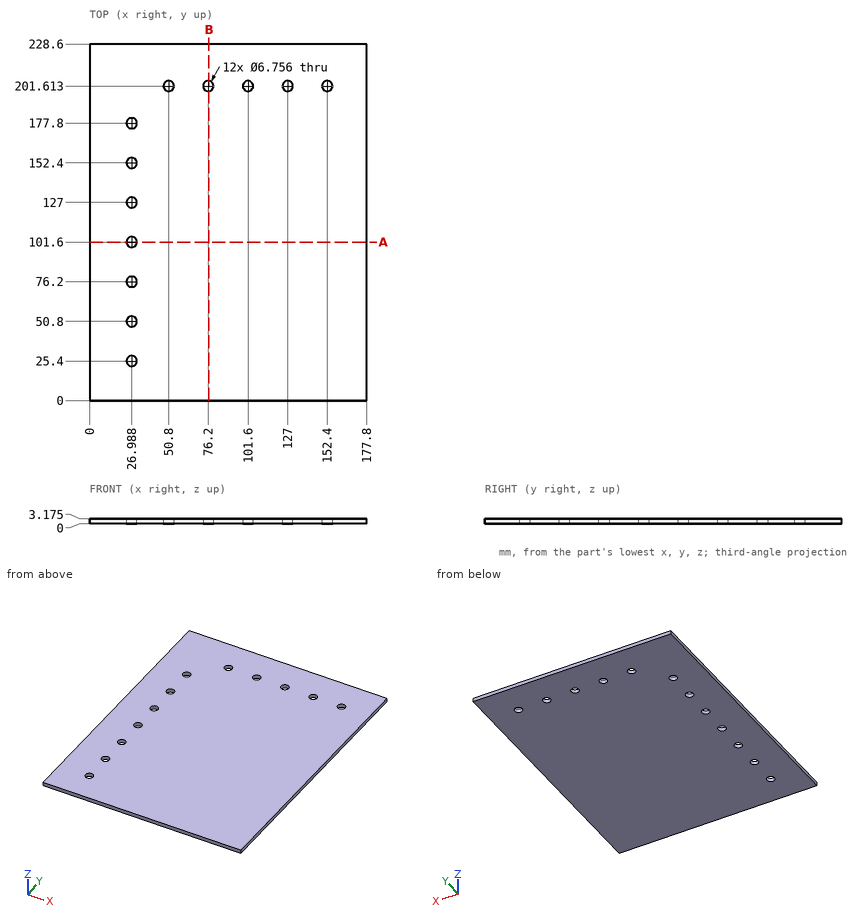
For this review, use the dimensioned drawing (mm, ordinates from the lowest corner) and the shaded views. Give positions to 0.01 mm unless a question says otherwise; leave off trailing zeros. Write each loop counter-clockwise with the first axis right and the second up, starting at its lowest first coordinate (ties: lowest second). Pieces come first, ordered by that corner, then holes.
(1) Consider section B-B, the plane x = 76.5. Give the boundary of the cut face in (y, z) (1 decimal).
(2) For P1, Ø11, axis at x = 152.4, y = 201.61, coming from the +Z side (1 decimal), flat-tipped, find the tip position at first contact; note if it passes through.
(3) To check wall thickness, follow L1, parallel to X at y = 202, z = 1.4 (1 decimal); L2, parallel to Y at x = 101.6, z = 2.45 (1 decimal); L3, parallel to Y at x = 52.5, z = 1 (1 decimal). State the ranges of each line that lie inside material, in increasing order.
(4) Consider section A-A, the plane y = 101.6. Give the boundary of the cut face in (x, z) (1 decimal).
Returned:
1. outline: (0, 0) - (198.2, 0) - (198.2, 3.2) - (0, 3.2) - close; (205, 0) - (228.6, 0) - (228.6, 3.2) - (205, 3.2) - close
2. P1: stops at z = 3.2
3. L1: x = 0 to 47.4, 54.2 to 72.8, 79.6 to 98.2, 105 to 123.6, 130.4 to 149, 155.8 to 177.8
3. L2: y = 0 to 198.2, 205 to 228.6
3. L3: y = 0 to 198.7, 204.5 to 228.6
4. outline: (0, 0) - (23.6, 0) - (23.6, 3.2) - (0, 3.2) - close; (30.4, 0) - (177.8, 0) - (177.8, 3.2) - (30.4, 3.2) - close
